from build123d import *

# Parameters (mm, degrees)
F0_W     = 152.4
F0_H     = 152.4
F1_DEPTH = 152.4
F2_W     = 116.84
F2_H     = 116.84
F3_DEPTH = 152.401
F4_W     = 116.84
F4_H     = 116.84
F5_DEPTH = 152.401
F6_W     = 116.84
F6_H     = 116.84
F7_DEPTH = 17.78
F8_SIZE  = 5.08


with BuildPart() as f1:
    # F0 (on Top) → F1 (new body)
    with BuildSketch(Plane.XY):
        with Locations((-76.2, 76.2)):
            Rectangle(F0_W, F0_H)
    extrude(amount=F1_DEPTH)

    # F2 (on face) → F3 (cut, through all)
    with BuildSketch(Plane.XZ):
        with Locations((-76.2, 76.2)):
            Rectangle(F2_W, F2_H)
    extrude(amount=-F3_DEPTH, mode=Mode.SUBTRACT)

    # F4 (on face) → F5 (cut, through all)
    with BuildSketch(Plane.YZ):
        with Locations((76.2, 76.2)):
            Rectangle(F4_W, F4_H)
    extrude(amount=-F5_DEPTH, mode=Mode.SUBTRACT)

    # F6 (on face) → F7 (cut)
    with BuildSketch(Plane.XY.offset(152.4)):
        with Locations((-76.2, 76.2)):
            Rectangle(F6_W, F6_H)
    extrude(amount=-F7_DEPTH, mode=Mode.SUBTRACT)

    # F8
    f8_edges = [f1.edges().sort_by_distance(p)[0] for p in [
        (-76.2, 0, 152.4),
        (0, 76.2, 152.4),
        (0, 0, 76.2),
        (-76.2, 152.4, 152.4),
        (-152.4, 76.2, 152.4),
        (0, 152.4, 76.2),
        (-152.4, 152.4, 76.2),
        (-152.4, 0, 76.2),
        (-76.2, 0, 0),
        (0, 76.2, 0),
        (-76.2, 152.4, 0),
        (-152.4, 76.2, 0),
    ]]
    chamfer(f8_edges, length=F8_SIZE)


solid = f1.part
Geometry: final body of the model. Coordinates: model frame, mm. A direction names the side the tool comes from. Give positions to 0.01 mm unless a question says otherwise; leave off trailing zeros. Loops run counter-clockwise (first coordinate to the right, second up) from the corner with the lowest first, then second, coordinate; pieces in that order, holes last. Notation, with made-up numbers: (4, 31) - (18, 31) arc R24 ccw to (18, 57) - close; hole circle Ø9 at (22, 16). An arc over 180 degrees is marked (long way). One line per question, with ' | ' between items. Start each with the question number.
(1) Ray query, line 1 (X direction, y = 137, z = 100); line 2 (Z direction, x = -108, y = 16). Return the intervals inside material, ascending. Write a range as from..to.
(2) Section query D-D on z = 42. Return loops of the section in (x, y), then the cut area to 3 significant figures.
(3) Contact query for a flat-ended pin moving along its axis: pin 1 (9 mm diameter, centred on x = -147.5, y = 53.5, fed in from -Z). Output: stop coordinate, or through.
(4) Section query A-A on x = -71. Return loops of the section in (y, z).
(5) Pull-direction query (Y, two-part tool) for faces 1 (the flat face through (-17.78, 143, 75)), 2 (the flat face through (-143, 134.62, 75)), 3 (the flat face through (-149.26, 3.55, 148.93)); classes: released by +Y, released by -Y, zero draft, split by the parting line, or undercut.
(6) Reachability of faces 4 (the flat face through (-17.78, 9, 75)), 5 (the flat face through (-77, 77, 0)), 6 (the flat face through (-75, 75, 17.78)), 7 (the flat face through (-17.78, 75, 144)), 8 (the flat face through (-140, 0, 75)) from +Z, -Z, +X, -X, +Y, -Y: full face, straight path, thin tool, end or side. Return the list, or none.
(7) Section query B-B on z = 141.5. Return loops of the section in (x, y), then the cut area to 3 significant figures.
The answers:
1) line 1: -152.4..-134.62, -17.78..0 | line 2: 0..17.78, 134.62..152.4
2) outline: (-152.4, 5.08) - (-147.32, 0) - (-134.62, 0) - (-134.62, 17.78) - (-152.4, 17.78) - close; (-152.4, 134.62) - (-134.62, 134.62) - (-134.62, 152.4) - (-147.32, 152.4) - (-152.4, 147.32) - close; (-17.78, 0) - (-5.08, 0) - (0, 5.08) - (0, 17.78) - (-17.78, 17.78) - close; (-17.78, 134.62) - (0, 134.62) - (0, 147.32) - (-5.08, 152.4) - (-17.78, 152.4) - close | area: 1,210 mm2
3) pin 1: z = 0
4) outline: (0, 5.08) - (5.08, 0) - (147.32, 0) - (152.4, 5.08) - (152.4, 17.78) - (0, 17.78) - close; (0, 134.62) - (17.78, 134.62) - (17.78, 152.4) - (5.08, 152.4) - (0, 147.32) - close; (134.62, 134.62) - (152.4, 134.62) - (152.4, 147.32) - (147.32, 152.4) - (134.62, 152.4) - close
5) face 1: zero draft | face 2: undercut | face 3: released by -Y
6) face 4: +Y, -Y | face 5: -Z, +X, -X, +Y, -Y | face 6: none | face 7: +Z | face 8: +Z, -Z, +X, -X, -Y
7) outline: (-152.4, 5.08) - (-147.32, 0) - (-5.08, 0) - (0, 5.08) - (0, 147.32) - (-5.08, 152.4) - (-147.32, 152.4) - (-152.4, 147.32) - close; hole (-134.62, 17.78) - (-17.78, 17.78) - (-17.78, 134.62) - (-134.62, 134.62) - close | area: 9,520 mm2
